Check sheet for the drawn part. Datum: minimum x, y, z corner. Units: mm. A direction names the side the tool comes from. Coordinates: 2 decimals unless noted, no trailing zeros. Write each loop counter-clockwise with the first axis right and the second up, starting at its lowest first coordinate (ties: lowest second). Pieces come first, ordered by that corner, then holes. Notation, with made-up numbers: M 81.25,-36.5 L 137.25,-36.5 A15 cw 137.25,-31.5 Z; hole C 41,61.25 d11. An arc over 180 degrees is marked long. Write item = value, one per line. Start each with the question number.
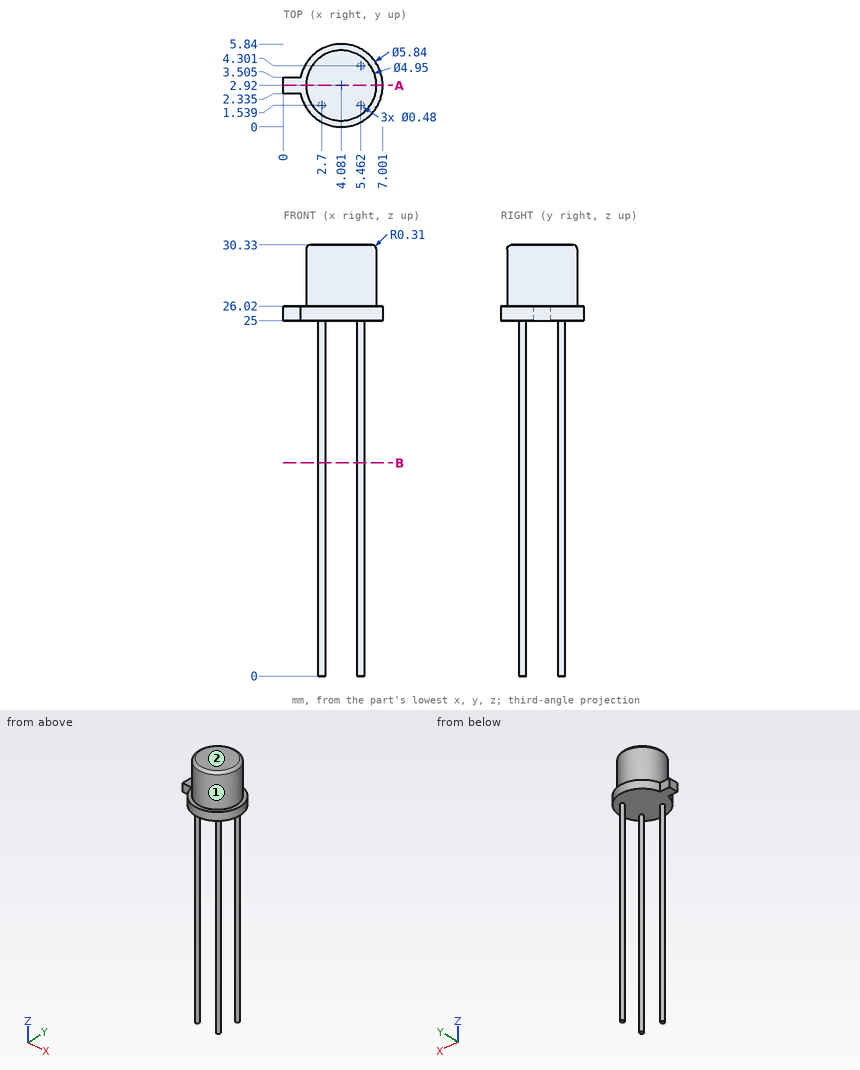
Q1. Gauge pin test, flat ends, axial feed: pin 1 (1.5 mm diameter, centred on y = 3.5, z = 14.5, fed in from -X); pin 2 (0.5 mm diameter, centred on x = 0.5, z = 25.5, fed in from +Y) (3 decimals); pin 3 (2 mm diameter, centred on x = 4, y = 2.5, fed in from -Z). Record the tip position at first contact, or that the pin passes through.
Q2. Cross-section at B-B on z = 15. Enter the section's corners in (x, y).
Q3. Cross-section at A-A on y = 2.92. Enter the section's corners in (x, z) (1 decimal).
Q4. Scan lines: L1, parallel to X at y = 1.55, z = 22; L2, parallel to Y at x = 5.5, z = 23 (1 decimal); L3, parallel to Z at x = 2.25, y = 1.9. Record each from-to range of solid material in increasing order.
Q5. Set-up check for the marked faces 1 and 2: record each of +Z, -Z, +X, -X, +Y, -Y from which the full face is reachable in a straight line by a thin tool's end or side.
Values found:
q1.pin_1 = 5.23
q1.pin_2 = 3.505
q1.pin_3 = 25
q2.outline = C 2.7,1.54 d0.48; C 5.46,1.54 d0.48; C 5.46,4.3 d0.48
q3.outline = M 0,25 L 7,25 L 7,26 L 6.6,26 L 6.6,30 A0.3 ccw 6.2,30.3 L 1.9,30.3 A0.3 ccw 1.6,30 L 1.6,26 L 0,26 Z
q4.L1 = 2.46 to 2.94, 5.22 to 5.7
q4.L2 = 1.3 to 1.8, 4.1 to 4.5
q4.L3 = 25 to 30.33
q5.face_1 = +Z
q5.face_2 = +Z, +X, -X, +Y, -Y
